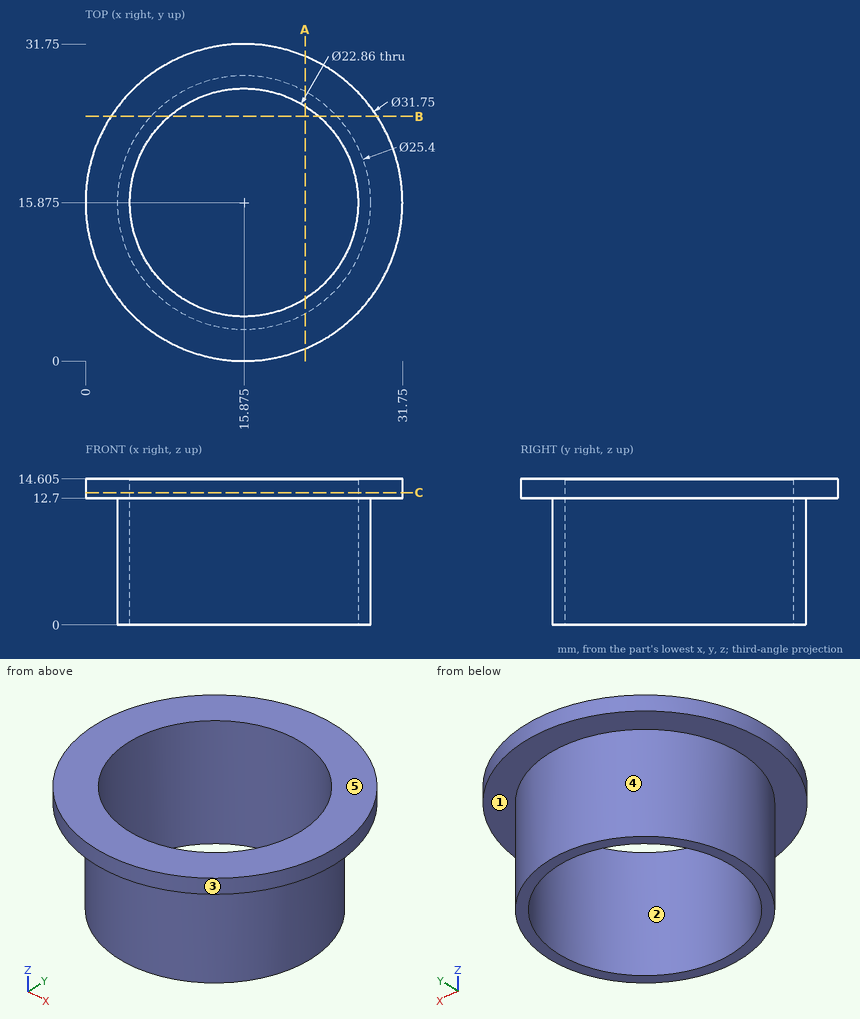
Can you work these out from the drawing? Everything is in mm from the part's minimum corner. A direction names the side the tool comes from. Coordinates: 2 decimals unless noted, no trailing zeros. Order: outer loops, then holes, each group sorted by start corner. A loop starts at its lowest first (then second) coordinate and runs counter-clockwise, first axis right, second up. Notation, with made-up numbers: (-23.75, 26) -> (17.25, 26) arc R25 ccw to (17.25, 61) -> close; hole circle Ø10 at (-7.5, 59). An arc over 180 degrees is marked (long way). Return JSON: item names as keys, results as strings.
1) If we section it at C-C on z = 13.25: List the corners of the cut face in (x, y) for me (3 decimals).
Conclusion:
{"outline": "circle Ø31.75 at (15.875, 15.875); hole circle Ø22.86 at (15.875, 15.875)"}
2) If I drill on probe 1 along Y at (x, z) = (16, 13.75); probe 2 along Z at (x, y) = (7.5, 4.5) (3 decimals); probe 3 along X at (y, z) = (18, 9.75), over which ranges is the centre line in solid material (lowest first)?
Conclusion:
{"probe 1": "y = 0 to 4.45, 27.3 to 31.75", "probe 2": "z = 12.7 to 14.605", "probe 3": "x = 3.35 to 4.64, 27.11 to 28.4"}
3) On a 3-axis mill with a long thin cutter (end or side, diameter ignored), from which of +Z, -Z, +X, -X, +Y, -Y can I reach the whole of each face in a straight line? I mean the marked faces 4 and 5. Say none if no direction works.
Conclusion:
{"face 4": "-Z", "face 5": "+Z, +X, -X, +Y, -Y"}
4) Thinking about a two-plate mould opening in Y: for the marked faces 1, 2 and 3, which applies, +Y half, -Y half, draft (parallel to the pull), parting line (faces both ways), or undercut?
Conclusion:
{"face 1": "draft", "face 2": "undercut", "face 3": "parting line"}
5) If we section it at B-B on y = 24.5: List the corners of the cut face in (x, z) for me (3 decimals), plus the area to 3 significant figures.
Conclusion:
{"outline": "(2.547, 12.7) -> (6.553, 12.7) -> (6.553, 0) -> (8.375, 0) -> (8.375, 14.605) -> (2.547, 14.605) -> close; (23.375, 0) -> (25.197, 0) -> (25.197, 12.7) -> (29.203, 12.7) -> (29.203, 14.605) -> (23.375, 14.605) -> close", "area": "68.5 mm²"}
6) I'm going to push flat-ended pins straight in: P1, Ø2, axis at y = 11, z = 4.5, coming from the +X side; P2, Ø1, axis at y = 26.5, z = 3.5, coming from the -X side; P3, Ø3, axis at y = 11.5, z = 10, coming from the -X side. Where does each tip first touch, or does it pass through?
Conclusion:
{"P1": "stops at x = 27.97", "P2": "stops at x = 8.21", "P3": "stops at x = 3.5"}
7) If we section it at A-A on x = 22: List the corners of the cut face in (y, z) for me (3 decimals), plus the area to 3 significant figures.
Conclusion:
{"outline": "(1.229, 12.7) -> (4.75, 12.7) -> (4.75, 0) -> (6.225, 0) -> (6.225, 14.605) -> (1.229, 14.605) -> close; (25.525, 0) -> (27, 0) -> (27, 12.7) -> (30.521, 12.7) -> (30.521, 14.605) -> (25.525, 14.605) -> close", "area": "56.5 mm²"}
